Design review of the part built by this model. Coordinates are the model's own, in mm. Round coordinates to 2 decimals unless told otherwise and drop trailing zeros. Loops run counter-clockwise (first coordinate to the right, second up) from the corner with the lowest first, then second, coordinate; pieces in that order, holes last. Notation, with made-up numbers: M 15.5,39 L 23.5,39 A15 ccw 23.5,63 Z; hole C 24,-16 d7. An arc over 180 degrees is marked long. Use a Markdown table: item, result.
Autodesk Inventor part; units mm, degrees
ref_plane "YZ Plane" through (0, 0, 0) normal (1, 0, 0) x (0, 1, 0)
ref_plane "XZ Plane" through (0, 0, 0) normal (0, 1, 0) x (-1, 0, 0)
ref_plane "XY Plane" through (0, 0, 0) normal (0, 0, 1) x (1, 0, 0)
sketch "Sketch1" plane through (0, 0, 0) normal (0, 1, 0) x (-1, 0, 0)
  line L0 (190, 210) -> (190, -210)
  line L1 (190, -210) -> (-150, -210)
  line L2 (-150, -210) -> (-150, 210)
  line L3 (-130, -190) -> (170, -190)
  line L4 (170, -190) -> (170, 190)
  line L5 (-130, 190) -> (-130, -190)
  line L6 (-140, -200) -> (180, -200)
  line L7 (180, -200) -> (180, 200)
  line L8 (-140, 200) -> (-140, -200)
  line L9 (190, -210) -> (190, -90)
  line L10 (190, -90) -> (-150, -90)
  line L11 (170, 190) -> (170, 210)
  line L12 (180, 200) -> (180, 210)
  line L13 (-130, 190) -> (-130, 210)
  line L14 (-140, 200) -> (-140, 210)
  line L15 (-150, 210) -> (-130, 210)
  line L16 (170, 210) -> (190, 210)
  line L17 (190, -90) -> (190, -100)
  line L18 (190, -100) -> (-150, -100)
  line L19 (190, -100) -> (190, -110)
  line L20 (190, -110) -> (-150, -110)
  circle A0 centre (180, 200) radius 2.5
  circle A1 centre (-140, 200) radius 2.5
  circle A2 centre (180, -100) radius 2.5
  circle A3 centre (-140, -100) radius 2.5
  circle A4 centre (20, -100) radius 2.5
  circle A5 centre (180, 100) radius 2.5
  circle A6 centre (180, 0) radius 2.5
  line L21 (0, 0) -> (0, 25.5231)
  circle A7 centre (20, -200) radius 2.5
  circle A8 centre (160, -200) radius 2.5
  line L22 (-140, -200) -> (-120, -200)
  circle A9 centre (-120, -200) radius 2.5
  circle A10 centre (-140, 0) radius 2.5
  circle A11 centre (-140, 100) radius 2.5
  point P0 (170, -90)
  point P1 (-130, -90)
  dimension "d0" = 340
  dimension "d1" = 420
  dimension "d2" = 20
  dimension "d3" = 10
  dimension "d4" = 120
  dimension "d5" = 10
  dimension "d6" = 10
  dimension "d7" = 5
  dimension "d8" = 5
  dimension "d9" = 5
  dimension "d10" = 5
  dimension "d11" = 5
  dimension "d12" = 5
  dimension "d13" = 5
  dimension "d14" = 5
  dimension "d15" = 5
  dimension "d25" = 320
  dimension "d26" = 300
  dimension "d27" = 20
  dimension "d28" = 5
  dimension "d29" = 5
  dimension "d30" = 5
extrude "Extrusion1" add sketch "Sketch1" along normal blind 3 contours L0 L10 L7 A6 A5 A0 L12 L16 | L0 L18 A2 L7 L10 | L12 A0 L7 A5 A6 L10 L4 L11 L16 | L0 L20 L7 A2 L18 | L7 A2 L18 L4 L10 | L0 L1 L2 L20 L8 L6 A9 A7 A8 L7 | L4 L18 A4 L5 L10 | L20 L4 L18 A2 L7 | L7 L6 A8 A7 A9 L8 L20 L5 L3 L4 | L4 L20 L5 L18 A4 | L10 L8 A10 A11 A1 L14 L15 L13 L5 | L5 L18 A3 L8 L10 | L4 L3 L5 L20 | L5 L20 L8 A3 L18 | L10 L2 L15 L14 A1 L8 A11 A10 | L8 A3 L18 L2 L10 | L2 L18 A3 L8 L20 | A10 L8 | L8 A10 | A11 L8 | L8 A11 | A9 L6 | L6 A9
sketch "Sketch2" plane through (0, 3, 0) normal (0, 1, 0) x (1, 0, 0)
  line L0 (130, 90) -> (130, -210)
  line L1 (130, -210) -> (150, -210)
  line L2 (150, -210) -> (150, 210)
  line L3 (150, 210) -> (-190, 210)
  line L4 (-190, 210) -> (-190, -210)
  line L5 (-190, -210) -> (-170, -210)
  line L6 (-170, -210) -> (-170, 90)
  line L7 (-170, 90) -> (130, 90)
  circle A0 centre (-180, -200) radius 2.5
  circle A1 centre (-180, -100) radius 2.5
  circle A2 centre (-180, 0) radius 2.5
  circle A3 centre (140, 100) radius 2.5
  circle A4 centre (140, -200) radius 2.5
  circle A5 centre (-20, 100) radius 2.5
  circle A6 centre (-20, 200) radius 2.5
  circle A7 centre (-160, 200) radius 2.5
  circle A8 centre (-180, 100) radius 2.5
  line L8 (-190, 210) -> (-170, 210)
  line L9 (-170, 210) -> (-170, 190)
  line L10 (-170, 190) -> (-190, 190)
  line L11 (-190, 190) -> (-190, 210)
  line L12 (150, 210) -> (130, 210)
  line L13 (130, 210) -> (130, 190)
  line L14 (130, 190) -> (150, 190)
  line L15 (150, 190) -> (150, 210)
  point P0 (0, 0)
  point P1 (150, 190)
  dimension "d19" = 20
  dimension "d20" = 20
  dimension "d21" = 20
  dimension "d22" = 20
extrude "Extrusion2" cut sketch "Sketch2" against normal blind 3 contours L14 L13 L3 L2 | L4 L3 L9 L10
extrude "Extrusion3" cut sketch "Sketch1" along normal blind 10 contours A10 L8 | L8 A10 | A11 L8 | L8 A11 | A9 L6 | L6 A9
properties part number "CaraMedia"
1. Take a section at C-C on x = -85.5. Give the boundary of the cut face in (y, z).
Check values:
| item | result |
|---|---|
| outline | M 0,-210 L 3,-210 L 3,-90 L 0,-90 Z |
2. Take a section at B-B on y = 0.85. Count the separate pieces of the cut face and the enclosed holes in it, and give its area (3 significant figures).
Check values:
| item | result |
|---|---|
| separate pieces | 1 |
| enclosed holes | 12 |
| area | 51,800 mm² |
3. Insertion check: pin 1 (1.5 mm diameter, centred on x = 144.5, y = 1.5, fed in from -Z); pin 2 (6.5 mm diameter, centred on x = 140, z = 200, fed in from +Y); pin 3 (1.5 mm diameter, centred on x = -106.5, y = 2.5, fed in from +Z). Each pin has a flat end and moves straight along its axis. Give the tip position at first contact, or say it passes through.
Check values:
| item | result |
|---|---|
| pin 1 | stops at z = -190 |
| pin 2 | stops at y = 3 |
| pin 3 | stops at z = -90 |
4. Take a section at A-A on z = 49. Give the boundary of the cut face in (x, y), and give its area (3 significant figures).
Check values:
| item | result |
|---|---|
| outline | M -190,0 L -170,0 L -170,3 L -190,3 Z; M 130,0 L 150,0 L 150,3 L 130,3 Z |
| area | 120 mm² |
5. Wall thickness on line 1 along Z through (x, y) = (-180, 1.9); line 2 along Z through (x, y) = (-20, 2.05); line 3 along X through (y, z) = (1.6, 100): over which ranges is each line inside the solid? List them lowest first. Write a range as from..to.
Check values:
| item | result |
|---|---|
| line 1 | z = -190..-102.5, -97.5..-2.5, 2.5..97.5, 102.5..197.5, 202.5..210 |
| line 2 | z = -210..-202.5, -197.5..-102.5, -97.5..-90 |
| line 3 | x = -190..-182.5, -177.5..-170, 130..137.5, 142.5..150 |
